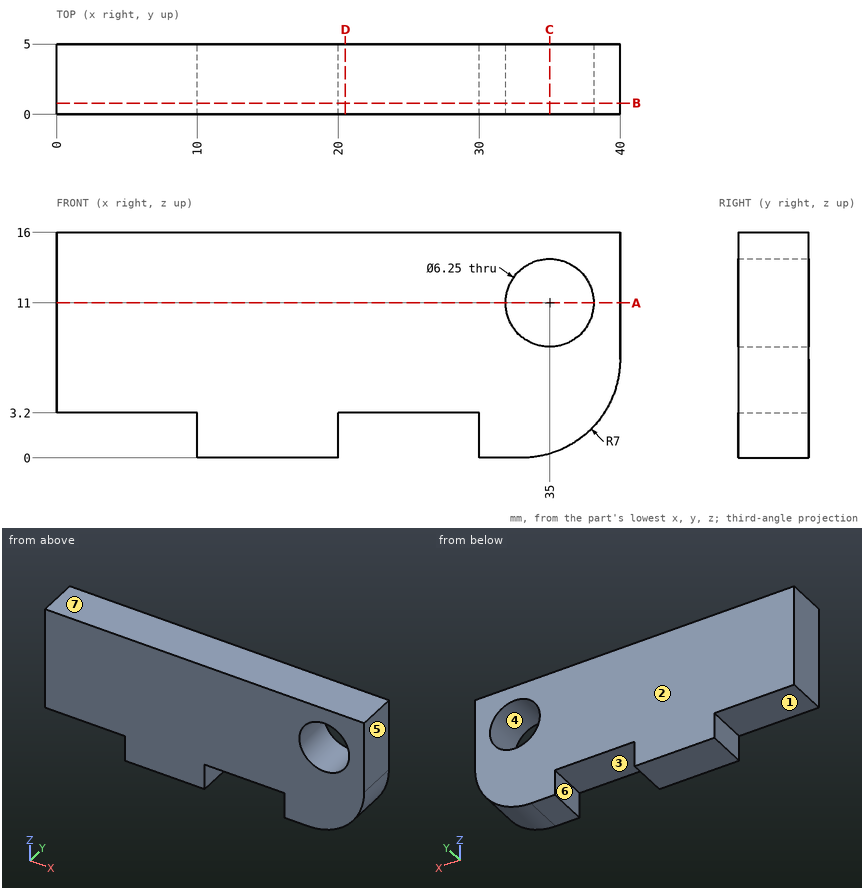
Source: three-view drawing plus pictorial views. Frame: mm from the lowest corner of the part. A direction names the side the tool comes from. Give positions to 0.01 mm unless a question says otherwise; leave off trailing zeros. Loops run counter-clockwise (first coordinate to the right, second up) from the corner with the lowest first, then second, coordinate; pieces in that order, holes last.
1) Section query B-B on y = 0.8. Return the cut outline in (x, z) (3 decimals).
A:
outline: (0, 3.2) - (10, 3.2) - (10, 0) - (20, 0) - (20, 3.2) - (30, 3.2) - (30, 0) - (33, 0) arc R7 ccw to (40, 7) - (40, 16) - (0, 16) - close; hole circle Ø6.25 at (35, 11)
2) Section query D-D on x = 20.5. Return the cut outline in (y, z).
A:
outline: (0, 3.2) - (5, 3.2) - (5, 16) - (0, 16) - close
3) Section query C-C on x = 35. Return the cut outline in (y, z) (3 decimals), and give its area (3 significant figures).
A:
outline: (0, 0.292) - (5, 0.292) - (5, 7.875) - (0, 7.875) - close; (0, 14.125) - (5, 14.125) - (5, 16) - (0, 16) - close
area: 47.3 mm2
4) Reachability of the marked faces 1, 2 and 3 from +Z, -Z, +X, -X, +Y, -Y: full face, straight path, thin tool, end or side. Return the list, or none.
A:
face 1: -Z, -X, +Y, -Y
face 2: +Z, -Z, +X, -X, +Y
face 3: -Z, +Y, -Y
5) Section query A-A on z = 11. Return the cut outline in (x, y) (3 decimals).
A:
outline: (0, 0) - (31.875, 0) - (31.875, 5) - (0, 5) - close; (38.125, 0) - (40, 0) - (40, 5) - (38.125, 5) - close
6) Contact query for flat-ended pins moving along their axis: pin 1 (2 mm diameter, centred on y = 1.5, z = 5, fed in from +X); pin 2 (1 mm diameter, centred on y = 2, z = 2, fed in from +X); pin 3 (1.5 mm diameter, centred on x = 7.5, y = 1.5, fed in from -Z). Output: stop coordinate, or through.
A:
pin 1: stops at x = 39.93
pin 2: stops at x = 38.36
pin 3: stops at z = 3.2
7) Line query: L1, parallel to X at y = 1.65, z = 11 (3 decimals); L2, parallel to X at y = 2.05, z = 8.5 (3 decimals); L3, parallel to Z at x = 35, y = 1.8 (3 decimals). Output: solid intervals per line, ascending.
A:
L1: x = 0 to 31.875, 38.125 to 40
L2: x = 0 to 33.125, 36.875 to 40
L3: z = 0.292 to 7.875, 14.125 to 16
8) Mould query, pull axis X, two halves, no side actions, for the marked faces 4, 5, 6 and 7. Classes: released by +X, released by -X, zero draft, split by the parting line, or undercut.
A:
face 4: undercut
face 5: released by +X
face 6: undercut
face 7: zero draft
